The listing builds one solid part. Answer for the finished solid, in the listing's coordinates (mm). A direction names the side the tool comes from. Give positions to 0.01 mm unless a question says otherwise; leave off trailing zeros. Order: outer loops, then holes, each group sorted by start corner. A loop starts at its lowest first (then second) coordinate and runs counter-clockwise, first axis right, second up. Notation, with made-up numbers: (11.5, 9) - (60.5, 9) arc R18 ccw to (60.5, 40) - close; hole circle Ø1 at (8, -22.5). An arc over 180 degrees is marked (long way). Use a Markdown table: item, result. Add a question column.
1) Find section A-A, the plane y = 38.5. Determine the outline of the cut face in (x, z).
2) Straight lines are drawn through the part: line 1 (Y direction, x = 3, z = 3.4); line 2 (Y direction, x = -8, z = 3.2); line 3 (Y direction, x = 8, z = 0.35). For each, find the intervals that lie inside material, in ascending order.
3) Find section B-B, the plane x = 15. Determine the outline of the cut face in (y, z), plus the area to 3 significant figures.
4) Flat-ended cylindrical pins translate along their axes: pin 1 (1 mm diameter, centred on x = 12, z = 2, fed in from +Y); pin 2 (1.5 mm diameter, centred on y = 8.5, z = 2.5, fed in from -X); pin 3 (5 mm diameter, centred on x = 0, y = 42.5, fed in from +Z) (3 decimals). Find the tip coordinate at first contact, or state that the pin passes through.
5) The mould has two halves that part along Y. Classify faces 4 (the face through (-8.19, -3.73, 1.97)), 5 (the face through (19.943, 26.727, 2.028)), 6 (the face through (8, 13, 4)): released by +Y, released by -Y, zero draft, split by the parting line, or undercut.
6) For faces 1 (the face through (1.84, -10.47, 1.97)), 2 (the face through (-4.113, -9.801, 1.972)), 3 (the face through (-1.17, 10.59, 1.97)), determine the directions among +Z, -Z, +X, -X, +Y, -Y from which every point of the face is accessible in a straight line to the end or side of a thin tool.
from build123d import *

# Parameters (mm, degrees)
ESBO_O1_R                = 3.75
RESSALTO_EXTRUS_O1_DEPTH = 4
RESSALTO_EXTRUS_O2_DEPTH = 4
CORTE_EXTRUS_O1_DEPTH    = 2


with BuildPart() as part:
    # Esbo_o1 → Ressalto-extrus_o1 (new body)
    with BuildSketch(Plane.XY):
        with BuildLine():
            Line((5.428931338, 10.411256864), (4.040153116, 8.653603149))
            ThreePointArc((4.040153116, 8.653603149), (3.651813796, 8.395770502), (3.186165661, 8.417146095))
            ThreePointArc((3.186165661, 8.417146095), (2.535977815, 8.635323765), (1.871064211, 8.803358377))
            ThreePointArc((1.871064211, 8.803358377), (1.465141223, 9.040151498), (1.27980553, 9.472002324))
            Line((1.27980553, 9.472002324), (1.087391415, 11.684866251))
            ThreePointArc((1.087391415, 11.684866251), (0.855086446, 12.165243662), (0.362160028, 12.369575749))
            ThreePointArc((0.362160028, 12.369575749), (0.013315066, 12.374869163), (-0.335540479, 12.370326458))
            ThreePointArc((-0.335540479, 12.370326458), (-0.826548297, 12.16926195), (-1.061642754, 11.693608494))
            Line((-1.061642754, 11.693608494), (-1.279697998, 9.464145904))
            ThreePointArc((-1.279697998, 9.464145904), (-1.466994971, 9.037291191), (-1.870279627, 8.803525096))
            ThreePointArc((-1.870279627, 8.803525096), (-2.535208203, 8.635549743), (-3.185415492, 8.41743002))
            ThreePointArc((-3.185415492, 8.41743002), (-3.654919666, 8.397174533), (-4.044310156, 8.660270526))
            Line((-4.044310156, 8.660270526), (-5.402543773, 10.417823198))
            ThreePointArc((-5.402543773, 10.417823198), (-5.857682784, 10.696348844), (-6.382829142, 10.601747792))
            ThreePointArc((-6.382829142, 10.601747792), (-6.679158034, 10.41760107), (-6.970178022, 10.225173956))
            ThreePointArc((-6.970178022, 10.225173956), (-7.274536404, 9.790568861), (-7.215152773, 9.263322051))
            Line((-7.215152773, 9.263322051), (-6.19325404, 7.269889205))
            ThreePointArc((-6.19325404, 7.269889205), (-6.120043199, 6.809535782), (-6.332924348, 6.394847082))
            ThreePointArc((-6.332924348, 6.394847082), (-6.80148353, 5.894049694), (-7.230548283, 5.359027107))
            ThreePointArc((-7.230548283, 5.359027107), (-7.614569385, 5.088153986), (-8.084385943, 5.098964027))
            Line((-8.084385943, 5.098964027), (-10.177209485, 5.843194888))
            ThreePointArc((-10.177209485, 5.843194888), (-10.710679119, 5.831438844), (-11.101315158, 5.46793982))
            ThreePointArc((-11.101315158, 5.46793982), (-11.251045651, 5.152818244), (-11.391833292, 4.833600971))
            ThreePointArc((-11.391833292, 4.833600971), (-11.412910602, 4.303439334), (-11.077902766, 3.891996308))
            Line((-11.077902766, 3.891996308), (-9.140495683, 2.76749405))
            ThreePointArc((-9.140495683, 2.76749405), (-8.830020954, 2.419800875), (-8.784910335, 1.955850303))
            ThreePointArc((-8.784910335, 1.955850303), (-8.908335893, 1.281230512), (-8.980033083, 0.599170952))
            ThreePointArc((-8.980033083, 0.599170952), (-9.156647127, 0.163680499), (-9.557726315, -0.081227523))
            Line((-9.557726315, -0.081227523), (-11.720683094, -0.586606513))
            ThreePointArc((-11.720683094, -0.586606513), (-12.163110512, -0.884911785), (-12.295212049, -1.401900411))
            ThreePointArc((-12.295212049, -1.401900411), (-12.25080577, -1.747947966), (-12.196661982, -2.09260617))
            ThreePointArc((-12.196661982, -2.09260617), (-11.927766323, -2.550001774), (-11.423496904, -2.715010763))
            Line((-11.423496904, -2.715010763), (-9.185694531, -2.613560912))
            ThreePointArc((-9.185694531, -2.613560912), (-8.736529446, -2.738203711), (-8.447749362, -3.104115127))
            ThreePointArc((-8.447749362, -3.104115127), (-8.186854553, -3.738370305), (-7.878420829, -4.350917747))
            ThreePointArc((-7.878420829, -4.350917747), (-7.791554103, -4.812760389), (-7.996556113, -5.235629909))
            Line((-7.996556113, -5.235629909), (-9.542922635, -6.83016449))
            ThreePointArc((-9.542922635, -6.83016449), (-9.753840257, -7.320309176), (-9.585465989, -7.826647167))
            ThreePointArc((-9.585465989, -7.826647167), (-9.361021617, -8.093753047), (-9.129136671, -8.354425638))
            ThreePointArc((-9.129136671, -8.354425638), (-8.655640515, -8.593835336), (-8.142211489, -8.4600211))
            Line((-8.142211489, -8.4600211), (-6.314500268, -7.16482875))
            ThreePointArc((-6.314500268, -7.16482875), (-5.869251568, -7.026847967), (-5.428487655, -7.178545938))
            ThreePointArc((-5.428487655, -7.178545938), (-4.866104738, -7.571064963), (-4.275465628, -7.919620803))
            ThreePointArc((-4.275465628, -7.919620803), (-3.952697704, -8.26118386), (-3.896535847, -8.727756791))
            Line((-3.896535847, -8.727756791), (-4.335351667, -10.905193502))
            ThreePointArc((-4.335351667, -10.905193502), (-4.247794638, -11.431560125), (-3.832402205, -11.766488747))
            ThreePointArc((-3.832402205, -11.766488747), (-3.499179242, -11.869848724), (-3.16317497, -11.963773995))
            ThreePointArc((-3.16317497, -11.963773995), (-2.635410001, -11.909186901), (-2.275831457, -11.519034514))
            Line((-2.275831457, -11.519034514), (-1.438496786, -9.441314085))
            ThreePointArc((-1.438496786, -9.441314085), (-1.138527788, -9.084517642), (-0.685719474, -8.973839134))
            ThreePointArc((-0.685719474, -8.973839134), (-0.000401051, -8.999999991), (0.684919701, -8.973900211))
            ThreePointArc((0.684919701, -8.973900211), (1.141112287, -9.086739826), (1.440607019, -9.44888256))
            Line((1.440607019, -9.44888256), (2.248662823, -11.517900629))
            ThreePointArc((2.248662823, -11.517900629), (2.606895765, -11.913371507), (3.137422201, -11.970553289))
            ThreePointArc((3.137422201, -11.970553289), (3.473627818, -11.877351299), (3.807072434, -11.774708641))
            ThreePointArc((3.807072434, -11.774708641), (4.221544568, -11.44345577), (4.313108983, -10.920835859))
            Line((4.313108983, -10.920835859), (3.894219261, -8.720248907))
            ThreePointArc((3.894219261, -8.720248907), (3.953670521, -8.257917155), (4.274759795, -7.920001811))
            ThreePointArc((4.274759795, -7.920001811), (4.865429967, -7.571498612), (5.427847864, -7.179029709))
            ThreePointArc((5.427847864, -7.179029709), (5.87262719, -7.0273201), (6.320367336, -7.170054878))
            Line((6.320367336, -7.170054878), (8.118742756, -8.473755688))
            ThreePointArc((8.118742756, -8.473755688), (8.633915182, -8.612771611), (9.111137226, -8.374051741))
            ThreePointArc((9.111137226, -8.374051741), (9.343582589, -8.113878758), (9.56860124, -7.847256489))
            ThreePointArc((9.56860124, -7.847256489), (9.738188564, -7.344508289), (9.532667795, -6.855348982))
            Line((9.532667795, -6.855348982), (7.990548209, -5.230566315))
            ThreePointArc((7.990548209, -5.230566315), (7.790606374, -4.809486318), (7.878033033, -4.351619874))
            ThreePointArc((7.878033033, -4.351619874), (8.186521347, -3.739099922), (8.447472682, -3.104867999))
            ThreePointArc((8.447472682, -3.104867999), (8.739624454, -2.736775896), (9.19345568, -2.614785434))
            Line((9.19345568, -2.614785434), (11.411179228, -2.739253189))
            ThreePointArc((11.411179228, -2.739253189), (11.919727533, -2.577677583), (12.192130558, -2.118847933))
            ThreePointArc((12.192130558, -2.118847933), (12.247015907, -1.774307042), (12.292166761, -1.428355848))
            ThreePointArc((12.292166761, -1.428355848), (12.163026498, -0.913731319), (11.725671937, -0.61333724))
            Line((11.725671937, -0.61333724), (9.549934558, -0.080215876))
            ThreePointArc((9.549934558, -0.080215876), (9.15407975, 0.165922443), (8.980086447, 0.598370627))
            ThreePointArc((8.980086447, 0.598370627), (8.908450044, 1.280436574), (8.78508461, 1.955067363))
            ThreePointArc((8.78508461, 1.955067363), (8.831852706, 2.422675318), (9.147686805, 2.77065991))
            Line((9.147686805, 2.77065991), (11.080646922, 3.864942843))
            ThreePointArc((11.080646922, 3.864942843), (11.421110614, 4.275810864), (11.402208583, 4.809075122))
            ThreePointArc((11.402208583, 4.809075122), (11.262108208, 5.128594624), (11.113056187, 5.444037682))
            ThreePointArc((11.113056187, 5.444037682), (10.726189458, 5.807148888), (10.195858089, 5.823404741))
            Line((10.195858089, 5.823404741), (8.077284162, 5.095602537))
            ThreePointArc((8.077284162, 5.095602537), (7.611197484, 5.088652), (7.231025864, 5.358382681))
            ThreePointArc((7.231025864, 5.358382681), (6.802008795, 5.893443506), (6.333494247, 6.394282651))
            ThreePointArc((6.333494247, 6.394282651), (6.120030126, 6.812944237), (6.197592003, 7.27644031))
            Line((6.197592003, 7.27644031), (7.232087511, 9.242046831))
            ThreePointArc((7.232087511, 9.242046831), (7.296371772, 9.771759573), (6.992165948, 10.210150805))
            ThreePointArc((6.992165948, 10.210150805), (6.701560727, 10.403203734), (6.405628795, 10.587987714))
            ThreePointArc((6.405628795, 10.587987714), (5.883863054, 10.684300355), (5.428931338, 10.411256864))
        make_face()
        Circle(ESBO_O1_R, mode=Mode.SUBTRACT)
    extrude(amount=RESSALTO_EXTRUS_O1_DEPTH)

    # Esbo_o6 → Ressalto-extrus_o2 (add)
    with BuildSketch(Plane.XY.offset(4)):
        with BuildLine():
            Line((0, 12.37), (0, 9))
            ThreePointArc((0, 9), (6.887269468, 5.79357569), (8.867092658, -1.540995716))
            Line((8.867092658, -1.540995716), (12.192130558, -2.118847933))
            ThreePointArc((12.192130558, -2.118847933), (19.845997755, 27.157089417), (0, 50))
            ThreePointArc((0, 50), (7.793428176, 31.185), (0, 12.37))
        make_face()
    extrude(amount=-RESSALTO_EXTRUS_O2_DEPTH)

    # Esbo_o7 → Corte-extrus_o1 (cut)
    with BuildSketch(Plane.XY.offset(4)):
        with BuildLine():
            Line((-2.524504061, 2.772972998), (9.641514463, 13.848869949))
            ThreePointArc((9.641514463, 13.848869949), (13.040353105, 13.81843663), (13.267495019, 10.427059792))
            Line((13.267495019, 10.427059792), (2.914466774, -2.359742237))
            ThreePointArc((2.914466774, -2.359742237), (-2.573753902, -2.727323019), (-2.524504061, 2.772972998))
        make_face()
    extrude(amount=-CORTE_EXTRUS_O1_DEPTH, mode=Mode.SUBTRACT)


solid = part.part
The answers:
| question | item | result |
|---|---|---|
| 1 | outline | (6.77, 0) - (14.74, 0) - (14.74, 4) - (6.77, 4) - close |
| 2 | line 1 | -11.99 to -2.25, 7.8 to 15.95, 46.42 to 48.66 |
| 2 | line 2 | -8.36 to -5.24, -4.12 to 5.07 |
| 2 | line 3 | -8.39 to -5.24, -4.12 to 45.5 |
| 3 | outline | (1.41, 0) - (38.13, 0) - (38.13, 4) - (1.41, 4) - close |
| 3 | area | 147 mm2 |
| 4 | pin 1 | y = 42.4 |
| 4 | pin 2 | x = -7.21 |
| 4 | pin 3 | through |
| 5 | face 4 | undercut |
| 5 | face 5 | split by the parting line |
| 5 | face 6 | zero draft |
| 6 | face 1 | +Z, -Z, -Y |
| 6 | face 2 | +Z, -Z, -X |
| 6 | face 3 | +Z, -Z, +Y |
